The model under review builds one solid part; all positions refer to its coordinate system, in mm. Face numbers are marked on the shaded views. A direction names the side the tool comes from. Round coordinates to 2 decimals unless told otherwise and drop trailing zeros. Order: outer loops, then holes, each group sorted by start corner. A loop starts at its lowest first (then second) coordinate and runs counter-clockwise, first axis right, second up. Notation, with made-up numbers: M -30.75,-20.75 L -19.75,-20.75 A15 ccw -19.75,-13.75 Z; hole C -1.75,-5 d9. An arc over 180 degrees is marked long. Use a Markdown table: item, result. Add a question column.
1. Consider section A-A on x = 18. State the section outline as (y, z) points, then the cut area to 3 significant figures.
2. Consider section D-D on x = 56.25. State the section outline as (y, z) points, then the cut area to 3 significant figures.
3. Consider section C-C on z = 0.25. State the section outline as (x, y) points.
4. The part is to be moulded in two halves that separate along X. For the marked faces 1 and 2, say which applies: +X half, -X half, draft (parallel to the pull), parting line (faces both ways), or undercut.
5. To check wall thickness, follow probe 1 along Y at (x, z) = (30, -11.9); probe 2 along Y at (x, z) = (55, -7). State the ranges of each line that lie inside material, in increasing order.
6. For the marked faces 3, 4 and 5, list the 3-axis set-ups (+Z, -Z, +X, -X, +Y, -Y) from which the entire face can be reached by the end or side of a thin tool; tool diameter is ignored.
7. Insertion check: P1, Ø5, axis at x = 55, y = 55, coming from the +Z side; P2, Ø1.6, axis at y = 56, z = -9, coming from the -X side; P3, Ø4, axis at x = 56.25, y = 30, coming from the -Z side; P4, Ø1.6, axis at x = 2.5, z = -9, coming from the -Y side. Each pin has a flat end and moves straight along its axis. Give the tip position at first contact, or say it passes through.
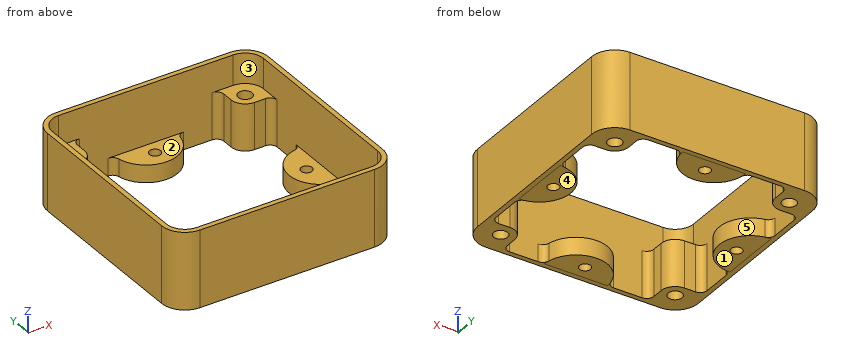
from build123d import *

# Parameters (mm, degrees)
BOSS_EXTRUDE1_DEPTH      = 7
BOSS_EXTRUDE1_DEPTH_BACK = 14.970201
BOSS_EXTRUDE2_START      = -14.970201
SKETCH2_R                = 2
BOSS_EXTRUDE2_DEPTH      = 13.350798149
BOSS_EXTRUDE3_START      = -14.970203
SKETCH3_R                = 1.6
BOSS_EXTRUDE3_DEPTH      = 5.000003
FILLET1_R                = 2


with BuildPart() as part:
    # Sketch1 → Boss-Extrude1 (new, two sides: drawn at the far end of the back side and taken through both)
    with BuildSketch(Plane.XY.offset(-BOSS_EXTRUDE1_DEPTH_BACK)):
        with BuildLine():
            Line((54.999742941, -1.649999966), (5.000257256, -1.649999966))
            ThreePointArc((5.000257256, -1.649999966), (0.297273819, 0.297273819), (-1.649999966, 5.000257256))
            Line((-1.649999966, 5.000257256), (-1.649999966, 54.999742941))
            ThreePointArc((-1.649999966, 54.999742941), (0.297274177, 59.702725823), (5.000257059, 61.649999966))
            Line((5.000257059, 61.649999966), (54.999743139, 61.649999966))
            ThreePointArc((54.999743139, 61.649999966), (59.702725466, 59.702725466), (61.649999966, 54.999743139))
            Line((61.649999966, 54.999743139), (61.649999966, 5.000257059))
            ThreePointArc((61.649999966, 5.000257059), (59.702725823, 0.297274177), (54.999742941, -1.649999966))
        make_face()
        with BuildLine():
            ThreePointArc((5.000039752, 60.249999994), (1.287223653, 58.712776347), (-0.249999994, 54.999960248))
            Line((-0.249999994, 54.999960248), (-0.249999994, 5.000039782))
            ThreePointArc((-0.249999994, 5.000039782), (1.287223296, 1.287223296), (5.000039782, -0.249999994))
            Line((5.000039782, -0.249999994), (54.999960248, -0.249999994))
            ThreePointArc((54.999960248, -0.249999994), (58.712776347, 1.287223653), (60.249999994, 5.000039752))
            Line((60.249999994, 5.000039752), (60.249999994, 54.999960279))
            ThreePointArc((60.249999994, 54.999960279), (58.712775989, 58.712775989), (54.999960279, 60.249999994))
            Line((54.999960279, 60.249999994), (5.000039752, 60.249999994))
        make_face(mode=Mode.SUBTRACT)
    extrude(amount=BOSS_EXTRUDE1_DEPTH + BOSS_EXTRUDE1_DEPTH_BACK)


with BuildPart() as boss_extrude2_tool:
    # Sketch2 → Boss-Extrude2 (new body)
    # profile 1 of 4: a face of its own
    with BuildSketch(Plane.XY.offset(BOSS_EXTRUDE2_START)):
        with BuildLine():
            Line((9.00000016, 54.99999922), (9.00000016, 60.249999994))
            Line((9.00000016, 60.249999994), (5.000039752, 60.249999994))
            add(Edge.make_bspline(
                [(-0.249999994, 54.999960248), (-0.250954892, 58.075921633), (1.924078367, 60.250954892), (5.000039752, 60.249999994)],
                knots=[0, 0, 0, 0, 1, 1, 1, 1], degree=3, weights=[1, 0.804591489, 0.804591489, 1]))
            Line((-0.249999994, 54.999960248), (-0.249999994, 50.99999922))
            Line((-0.249999994, 50.99999922), (5.00000016, 50.99999922))
            ThreePointArc((5.00000016, 50.99999922), (7.828427285, 52.171572095), (9.00000016, 54.99999922))
        make_face()
        with Locations(Location((5.00000016, 54.99999922, 0), (0, 0, 90))):
            Circle(SKETCH2_R, mode=Mode.SUBTRACT)
    # profile 2 of 4: a face of its own
    with BuildSketch(Plane.XY.offset(BOSS_EXTRUDE2_START)):
        with BuildLine():
            Line((50.99999922, 54.99999984), (50.99999922, 60.249999994))
            Line((50.99999922, 60.249999994), (54.999960248, 60.249999994))
            add(Edge.make_bspline(
                [(54.999960248, 60.249999994), (58.075921633, 60.250954892), (60.250954892, 58.075921633), (60.249999994, 54.999960248)],
                knots=[0, 0, 0, 0, 1, 1, 1, 1], degree=3, weights=[1, 0.804591489, 0.804591489, 1]))
            Line((60.249999994, 54.999960248), (60.249999994, 50.99999984))
            Line((60.249999994, 50.99999984), (54.99999922, 50.99999984))
            ThreePointArc((54.99999922, 50.99999984), (52.171572095, 52.171572715), (50.99999922, 54.99999984))
        make_face()
        with Locations(Location((54.99999922, 54.99999984, 0), (0, 0, 90))):
            Circle(SKETCH2_R, mode=Mode.SUBTRACT)
    # profile 3 of 4: a face of its own
    with BuildSketch(Plane.XY.offset(BOSS_EXTRUDE2_START)):
        with BuildLine():
            Line((54.99999984, 9.00000078), (60.249999994, 9.00000078))
            Line((60.249999994, 9.00000078), (60.249999994, 5.000039752))
            add(Edge.make_bspline(
                [(60.249999994, 5.000039752), (60.250954892, 1.924078367), (58.075921633, -0.250954892), (54.999960248, -0.249999994)],
                knots=[0, 0, 0, 0, 1, 1, 1, 1], degree=3, weights=[1, 0.804591489, 0.804591489, 1]))
            Line((54.999960248, -0.249999994), (50.99999984, -0.249999994))
            Line((50.99999984, -0.249999994), (50.99999984, 5.00000078))
            ThreePointArc((50.99999984, 5.00000078), (52.171572715, 7.828427905), (54.99999984, 9.00000078))
        make_face()
        with Locations(Location((54.99999984, 5.00000078, 0), (0, 0, 90))):
            Circle(SKETCH2_R, mode=Mode.SUBTRACT)
    # profile 4 of 4: a face of its own
    with BuildSketch(Plane.XY.offset(BOSS_EXTRUDE2_START)):
        with BuildLine():
            Line((9.00000078, 5.00000016), (9.00000078, -0.249999994))
            Line((9.00000078, -0.249999994), (5.000039752, -0.249999994))
            add(Edge.make_bspline(
                [(5.000039752, -0.249999994), (1.924078367, -0.250954892), (-0.250954892, 1.924078367), (-0.249999994, 5.000039752)],
                knots=[0, 0, 0, 0, 1, 1, 1, 1], degree=3, weights=[1, 0.804591489, 0.804591489, 1]))
            Line((-0.249999994, 5.000039752), (-0.249999994, 9.00000016))
            Line((-0.249999994, 9.00000016), (5.00000078, 9.00000016))
            ThreePointArc((5.00000078, 9.00000016), (7.828427905, 7.828427285), (9.00000078, 5.00000016))
        make_face()
        with Locations(Location((5.00000078, 5.00000016, 0), (0, 0, 90))):
            Circle(SKETCH2_R, mode=Mode.SUBTRACT)
    extrude(amount=BOSS_EXTRUDE2_DEPTH)


with BuildPart() as part_1:
    add(part.part)


with BuildPart() as part_2:
    # Boss-Extrude2: joined with boss_extrude2_tool
    add(part_1.part.fuse(boss_extrude2_tool.part, tol=0.00001))

    # Sketch3 → Boss-Extrude3 (add)
    # profile 1 of 4: a face of its own
    with BuildSketch(Plane.XY.offset(BOSS_EXTRUDE3_START)):
        with BuildLine():
            Line((60.249999994, 20.999999985), (60.249999994, 38.999999985))
            ThreePointArc((60.249999994, 38.999999985), (51.249999994, 29.999999985), (60.249999994, 20.999999985))
        make_face()
        with Locations(Location((56.249999994, 29.999999985, 0), (0, 0, 180))):
            Circle(SKETCH3_R, mode=Mode.SUBTRACT)
    # profile 2 of 4: a face of its own
    with BuildSketch(Plane.XY.offset(BOSS_EXTRUDE3_START)):
        with BuildLine():
            Line((39.000000015, 60.249999994), (21.000000015, 60.249999994))
            ThreePointArc((21.000000015, 60.249999994), (30.000000015, 51.249999994), (39.000000015, 60.249999994))
        make_face()
        with Locations(Location((30.000000015, 56.249999994, 0), (0, 0, 180))):
            Circle(SKETCH3_R, mode=Mode.SUBTRACT)
    # profile 3 of 4: a face of its own
    with BuildSketch(Plane.XY.offset(BOSS_EXTRUDE3_START)):
        with BuildLine():
            Line((20.999999985, -0.249999994), (38.999999985, -0.249999994))
            ThreePointArc((38.999999985, -0.249999994), (29.999999985, 8.750000006), (20.999999985, -0.249999994))
        make_face()
        with Locations(Location((29.999999985, 3.750000006, 0), (0, 0, 180))):
            Circle(SKETCH3_R, mode=Mode.SUBTRACT)
    # profile 4 of 4: a face of its own
    with BuildSketch(Plane.XY.offset(BOSS_EXTRUDE3_START)):
        with BuildLine():
            Line((-0.249999994, 39.000000015), (-0.249999994, 21.000000015))
            ThreePointArc((-0.249999994, 21.000000015), (8.750000006, 30.000000015), (-0.249999994, 39.000000015))
        make_face()
        with Locations(Location((3.750000006, 30.000000015, 0), (0, 0, 180))):
            Circle(SKETCH3_R, mode=Mode.SUBTRACT)
    extrude(amount=BOSS_EXTRUDE3_DEPTH)

    # Fillet1
    fillet1_edges = [part_2.edges().sort_by_distance(p)[0] for p in [
        (-0.249999994, 50.99999922, -8.294801925),
        (9.00000016, 60.249999994, -8.294801925),
        (50.99999922, 60.249999994, -8.294801925),
        (60.249999994, 50.99999984, -8.294801925),
        (60.249999994, 9.00000078, -8.294801925),
        (50.99999984, -0.249999994, -8.294801925),
        (9.00000078, -0.249999994, -8.294801925),
        (-0.249999994, 9.00000016, -8.294801925),
        (21.000000015, 60.249999994, -12.4702005),
        (39.000000015, 60.249999994, -12.4702005),
        (60.249999994, 38.999999985, -12.4702005),
        (60.249999994, 20.999999985, -12.4702005),
        (38.999999985, -0.249999994, -12.4702005),
        (20.999999985, -0.249999994, -12.4702005),
        (-0.249999994, 21.000000015, -12.4702005),
        (-0.249999994, 39.000000015, -12.4702005),
    ]]
    fillet(fillet1_edges, radius=FILLET1_R)


solid = part_2.part
Answer block:
| question | item | result |
|---|---|---|
| 1 | outline | M -1.65,-14.97 L -0.25,-14.97 L -0.25,7 L -1.65,7 Z; M 60.25,-14.97 L 61.65,-14.97 L 61.65,7 L 60.25,7 Z |
| 1 | area | 61.5 mm^2 |
| 2 | outline | M -1.53,-14.97 L 3.44,-14.97 L 3.44,-1.62 L -0.1,-1.62 L -0.1,7 L -1.53,7 Z; M 6.56,-14.97 L 9,-14.97 L 9,-1.62 L 6.56,-1.62 Z; M 21.94,-14.97 L 28.4,-14.97 L 28.4,-9.97 L 21.94,-9.97 Z; M 31.6,-14.97 L 38.06,-14.97 L 38.06,-9.97 L 31.6,-9.97 Z; M 51,-14.97 L 53.44,-14.97 L 53.44,-1.62 L 51,-1.62 Z; M 56.56,-14.97 L 61.53,-14.97 L 61.53,7 L 60.1,7 L 60.1,-1.62 L 56.56,-1.62 Z |
| 2 | area | 287 mm^2 |
| 3 | outline | M -1.65,5 A6.65 ccw 5,-1.65 L 55,-1.65 A6.65 ccw 61.65,5 L 61.65,55 A6.65 ccw 55,61.65 L 5,61.65 A6.65 ccw -1.65,55 Z; hole M -0.25,5 A5.25 ccw 5,-0.25 L 55,-0.25 A5.25 ccw 60.25,5 L 60.25,55 A5.25 ccw 55,60.25 L 5,60.25 A5.25 ccw -0.25,55 Z |
| 4 | face 1 | draft |
| 4 | face 2 | undercut |
| 5 | probe 1 | -1.65 to 2.15, 5.35 to 8.75, 51.25 to 54.65, 57.85 to 61.65 |
| 5 | probe 2 | -1.65 to 3, 7 to 9, 51 to 53, 57 to 61.65 |
| 6 | face 3 | +Z |
| 6 | face 4 | -Z, +X, -X, +Y, -Y |
| 6 | face 5 | +Z, -Z |
| 7 | P1 | z = -1.62 |
| 7 | P2 | x = -1.65 |
| 7 | P3 | z = -14.97 |
| 7 | P4 | y = -1.43 |
